Input: part model. Units: mm. Frame: model coordinates. A direction names the side the tool comes from. Coordinates: 2 decimals unless noted, no trailing zeros. Order: outer loops, then holes, each group sorted by start corner. A loop starts at its lowest first (then second) coordinate and runs counter-clockwise, first axis right, second up. Notation, with made-up numbers: (-5.5, -36) -> (9.5, -36) arc R31 ccw to (9.5, -2) -> close; hole circle Ø11 at (-7, 11). An arc over 180 degrees is marked (long way). Write each question's results on one line, items separated by ' | '.
```python
from build123d import *

# Parameters (mm, degrees)
F1_DEPTH = 12.7
F2_R     = 2.794
F3_DEPTH = 12.7


with BuildPart() as f1:
    # F0 (on Top) → F1 (new body)
    with BuildSketch(Plane.XY):
        with BuildLine():
            ThreePointArc((6.162883, -1.530153), (6.303047, -0.770776), (6.35, 0))
            ThreePointArc((6.35, 0), (6.345169, 0.247642), (6.330685, 0.494907))
            ThreePointArc((6.330685, 0.494907), (6.328312, 0.524379), (6.325801, 0.55384))
            ThreePointArc((6.325801, 0.55384), (6.155692, 1.558833), (5.826975, 2.523661))
            ThreePointArc((5.826975, 2.523661), (5.815161, 2.550766), (5.80322, 2.577815))
            ThreePointArc((5.80322, 2.577815), (5.316007, 3.473121), (4.691822, 4.278938))
            ThreePointArc((4.691822, 4.278938), (4.671847, 4.300738), (4.651771, 4.322445))
            ThreePointArc((4.651771, 4.322445), (3.900251, 5.011042), (3.048237, 5.570525))
            ThreePointArc((3.048237, 5.570525), (3.022266, 5.584658), (2.996229, 5.59867))
            ThreePointArc((2.996229, 5.59867), (2.061842, 6.005939), (1.074329, 6.25846))
            ThreePointArc((1.074329, 6.25846), (1.045176, 6.263394), (1.016, 6.268193))
            ThreePointArc((1.016, 6.268193), (0, 6.35), (-1.016, 6.268193))
            ThreePointArc((-1.016, 6.268193), (-1.045176, 6.263394), (-1.074329, 6.25846))
            ThreePointArc((-1.074329, 6.25846), (-2.061842, 6.005939), (-2.996229, 5.59867))
            ThreePointArc((-2.996229, 5.59867), (-3.022266, 5.584658), (-3.048237, 5.570525))
            ThreePointArc((-3.048237, 5.570525), (-3.900251, 5.011042), (-4.651771, 4.322445))
            ThreePointArc((-4.651771, 4.322445), (-4.671847, 4.300738), (-4.691822, 4.278938))
            ThreePointArc((-4.691822, 4.278938), (-5.316007, 3.473121), (-5.80322, 2.577815))
            ThreePointArc((-5.80322, 2.577815), (-5.815161, 2.550766), (-5.826975, 2.523661))
            ThreePointArc((-5.826975, 2.523661), (-6.155692, 1.558833), (-6.325801, 0.55384))
            ThreePointArc((-6.325801, 0.55384), (-6.328312, 0.524379), (-6.330685, 0.494907))
            ThreePointArc((-6.330685, 0.494907), (-6.328312, -0.524379), (-6.162883, -1.530153))
            ThreePointArc((-6.162883, -1.530153), (-6.155692, -1.558833), (-6.148367, -1.587479))
            ThreePointArc((-6.148367, -1.587479), (-5.815161, -2.550766), (-5.332121, -3.44833))
            ThreePointArc((-5.332121, -3.44833), (-5.316007, -3.473121), (-5.299778, -3.497836))
            ThreePointArc((-5.299778, -3.497836), (-4.671847, -4.300738), (-3.923541, -4.992827))
            ThreePointArc((-3.923541, -4.992827), (-3.900251, -5.011042), (-3.876875, -5.029149))
            ThreePointArc((-3.876875, -5.029149), (-3.022266, -5.584658), (-2.089785, -5.996274))
            ThreePointArc((-2.089785, -5.996274), (-2.061842, -6.005939), (-2.033854, -6.015475))
            ThreePointArc((-2.033854, -6.015475), (-1.045176, -6.263394), (-0.029568, -6.349931))
            ThreePointArc((-0.029568, -6.349931), (0, -6.35), (0.029568, -6.349931))
            ThreePointArc((0.029568, -6.349931), (1.045176, -6.263394), (2.033854, -6.015475))
            ThreePointArc((2.033854, -6.015475), (2.061842, -6.005939), (2.089785, -5.996274))
            ThreePointArc((2.089785, -5.996274), (3.022266, -5.584658), (3.876875, -5.029149))
            ThreePointArc((3.876875, -5.029149), (3.900251, -5.011042), (3.923541, -4.992827))
            ThreePointArc((3.923541, -4.992827), (4.671847, -4.300738), (5.299778, -3.497836))
            ThreePointArc((5.299778, -3.497836), (5.316007, -3.473121), (5.332121, -3.44833))
            ThreePointArc((5.332121, -3.44833), (5.815161, -2.550766), (6.148367, -1.587479))
            ThreePointArc((6.148367, -1.587479), (6.155692, -1.558833), (6.162883, -1.530153))
        make_face()
        with BuildLine():
            ThreePointArc((1.074329, 6.25846), (2.061842, 6.005939), (2.996229, 5.59867))
            Line((2.996229, 5.59867), (2.919235, 8.50344))
            Line((2.919235, 8.50344), (1.074329, 6.25846))
        make_face()
        with BuildLine():
            ThreePointArc((-6.325801, 0.55384), (-6.155692, 1.558833), (-5.826975, 2.523661))
            Line((-5.826975, 2.523661), (-8.715465, 2.207055))
            Line((-8.715465, 2.207055), (-6.325801, 0.55384))
        make_face()
        with BuildLine():
            ThreePointArc((-4.651771, 4.322445), (-3.900251, 5.011042), (-3.048237, 5.570525))
            Line((-3.048237, 5.570525), (-5.522125, 7.094826))
            Line((-5.522125, 7.094826), (-4.651771, 4.322445))
        make_face()
        with BuildLine():
            ThreePointArc((5.826975, 2.523661), (6.155692, 1.558833), (6.325801, 0.55384))
            Line((6.325801, 0.55384), (8.715465, 2.207055))
            Line((8.715465, 2.207055), (5.826975, 2.523661))
        make_face()
        with BuildLine():
            ThreePointArc((6.330685, 0.494907), (6.345169, 0.247642), (6.35, 0))
            ThreePointArc((6.35, 0), (6.303047, -0.770776), (6.162883, -1.530153))
            Line((6.162883, -1.530153), (8.959866, -0.742436))
            Line((8.959866, -0.742436), (6.330685, 0.494907))
        make_face()
        with BuildLine():
            Line((8.233328, -3.611472), (6.148367, -1.587479))
            ThreePointArc((6.148367, -1.587479), (5.815161, -2.550766), (5.332121, -3.44833))
            Line((5.332121, -3.44833), (8.233328, -3.611472))
        make_face()
        with BuildLine():
            Line((-4.27904, -7.906974), (-2.089785, -5.996274))
            ThreePointArc((-2.089785, -5.996274), (-3.022266, -5.584658), (-3.876875, -5.029149))
            Line((-3.876875, -5.029149), (-4.27904, -7.906974))
        make_face()
        with BuildLine():
            Line((-6.61458, -6.08915), (-3.923541, -4.992827))
            ThreePointArc((-3.923541, -4.992827), (-4.671847, -4.300738), (-5.299778, -3.497836))
            Line((-5.299778, -3.497836), (-6.61458, -6.08915))
        make_face()
        with BuildLine():
            Line((-8.959866, -0.742436), (-6.162883, -1.530153))
            ThreePointArc((-6.162883, -1.530153), (-6.328312, -0.524379), (-6.330685, 0.494907))
            Line((-6.330685, 0.494907), (-8.959866, -0.742436))
        make_face()
        with BuildLine():
            ThreePointArc((-5.80322, 2.577815), (-5.316007, 3.473121), (-4.691822, 4.278938))
            Line((-4.691822, 4.278938), (-7.526607, 4.917378))
            Line((-7.526607, 4.917378), (-5.80322, 2.577815))
        make_face()
        with BuildLine():
            ThreePointArc((-2.996229, 5.59867), (-2.061842, 6.005939), (-1.074329, 6.25846))
            Line((-1.074329, 6.25846), (-2.919235, 8.50344))
            Line((-2.919235, 8.50344), (-2.996229, 5.59867))
        make_face()
        with BuildLine():
            ThreePointArc((-1.016, 6.268193), (0, 6.35), (1.016, 6.268193))
            Line((1.016, 6.268193), (0, 8.990574))
            Line((0, 8.990574), (-1.016, 6.268193))
        make_face()
        with BuildLine():
            ThreePointArc((3.048237, 5.570525), (3.900251, 5.011042), (4.651771, 4.322445))
            Line((4.651771, 4.322445), (5.522125, 7.094826))
            Line((5.522125, 7.094826), (3.048237, 5.570525))
        make_face()
        with BuildLine():
            Line((1.4798, -8.867954), (2.033854, -6.015475))
            ThreePointArc((2.033854, -6.015475), (1.045176, -6.263394), (0.029568, -6.349931))
            Line((0.029568, -6.349931), (1.4798, -8.867954))
        make_face()
        with BuildLine():
            Line((-1.4798, -8.867954), (-0.029568, -6.349931))
            ThreePointArc((-0.029568, -6.349931), (-1.045176, -6.263394), (-2.033854, -6.015475))
            Line((-2.033854, -6.015475), (-1.4798, -8.867954))
        make_face()
        with BuildLine():
            Line((4.27904, -7.906974), (3.876875, -5.029149))
            ThreePointArc((3.876875, -5.029149), (3.022266, -5.584658), (2.089785, -5.996274))
            Line((2.089785, -5.996274), (4.27904, -7.906974))
        make_face()
        with BuildLine():
            Line((6.61458, -6.08915), (5.299778, -3.497836))
            ThreePointArc((5.299778, -3.497836), (4.671847, -4.300738), (3.923541, -4.992827))
            Line((3.923541, -4.992827), (6.61458, -6.08915))
        make_face()
        with BuildLine():
            ThreePointArc((4.691822, 4.278938), (5.316007, 3.473121), (5.80322, 2.577815))
            Line((5.80322, 2.577815), (7.526607, 4.917378))
            Line((7.526607, 4.917378), (4.691822, 4.278938))
        make_face()
        with BuildLine():
            Line((-8.233328, -3.611472), (-5.332121, -3.44833))
            ThreePointArc((-5.332121, -3.44833), (-5.815161, -2.550766), (-6.148367, -1.587479))
            Line((-6.148367, -1.587479), (-8.233328, -3.611472))
        make_face()
    extrude(amount=F1_DEPTH)

    # F2 (on face) → F3 (cut)
    with BuildSketch(Plane.XY.offset(12.7)):
        Circle(F2_R)
    extrude(amount=-F3_DEPTH, mode=Mode.SUBTRACT)


solid = f1.part
```
(1) Pin query (flat end, axial travel): P1, Ø2, axis at x = 6.5, z = 8.5, coming from the -Y side; P2, Ø5, axis at y = 1, z = 10, coming from the -X side; P3, Ø4, axis at y = 1.5, z = 4, coming from the +X side. Return the tip coordinate at first contact, or that it passes through.
Return value:
P1: y = -6.09 | P2: x = -8.96 | P3: x = 8.72
(2) Line query: line 1 along X through (y, z) = (-6.25, 3.5); line 2 along X through (y, z) = (-7.5, 9.75); line 3 along X through (y, z) = (-5.75, 4.75). Output: solid intervals per line, ascending. Write a range as from..to.
Return value:
line 1: -4.05..-2.38, -1.99..1.99, 2.38..4.05 | line 2: -4.22..-3.81, -1.75..-0.69, 0.69..1.75, 3.81..4.22 | line 3: -6.44..-5.78, -3.98..3.98, 5.78..6.44
(3) Cut plane A-A, the plane x = -0.5. Return loops of the section in (y, z), plus the area to 3 significant figures.
Return value:
outline: (-7.17, 0) -> (-2.75, 0) -> (-2.75, 12.7) -> (-7.17, 12.7) -> close; (2.75, 0) -> (7.65, 0) -> (7.65, 12.7) -> (2.75, 12.7) -> close | area: 118 mm2
(4) Reachability of faces 1 (the face through (7.205, -2.614, 6.261)), 2 (the face through (1.753, -7.462, 6.261)), 3 (the face through (-7.251, 2.368, 6.261)), 4 (the face through (2.01, 7.4, 6.26)), 5 (the face through (-6.089, 4.594, 6.261)) from +Z, -Z, +X, -X, +Y, -Y: full face, straight path, thin tool, end or side. Return the list, or none.
Return value:
face 1: +Z, -Z, +X | face 2: +Z, -Z, -Y | face 3: +Z, -Z, -X | face 4: +Z, -Z, +Y | face 5: +Z, -Z
(5) Mould query, pull axis X, two halves, no side actions, for faces 6 (the face through (7.291, 2.363, 6.261)), 7 (the face through (-7.58, -1.13, 6.26)), 8 (the face through (-0.5, 7.65, 6.26)). Classes: +X half, -X half, draft (parallel to the pull), parting line (faces both ways), or undercut.
Return value:
face 6: +X half | face 7: -X half | face 8: undercut
(6) Cut plane B-B, the plane y = 0. Return loops of the section in (x, z), plus the area to 3 significant figures.
Return value:
outline: (-7.38, 0) -> (-2.79, 0) -> (-2.79, 12.7) -> (-7.38, 12.7) -> close; (2.79, 0) -> (7.38, 0) -> (7.38, 12.7) -> (2.79, 12.7) -> close | area: 117 mm2
